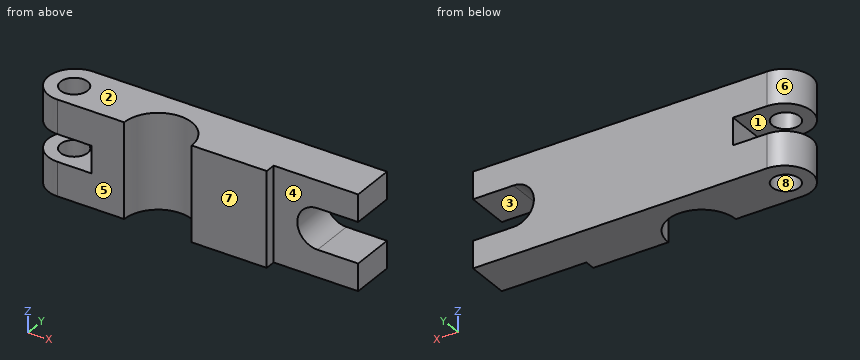
Autodesk Inventor part; units mm, degrees
ref_plane "YZ Plane" through (0, 0, 0) normal (1, 0, 0) x (0, 1, 0)
ref_plane "XZ Plane" through (0, 0, 0) normal (0, 1, 0) x (-1, 0, 0)
ref_plane "XY Plane" through (0, 0, 0) normal (0, 0, 1) x (1, 0, 0)
sketch "Szkic1" plane through (0, 0, 0) normal (0, 0, 1) x (1, 0, 0)
  line L0 (-28.581, 16.053) -> (52, 16.053)
  circle A0 centre (-35, 7.6573) radius 4
  line L1 (52, 16.053) -> (52, 3.053)
  line L2 (52, 3.053) -> (27, 3.053)
  line L3 (27, 3.053) -> (27, -0.0459)
  line L4 (27, -0.0459) -> (4.7982, -0.0459)
  arc A1 (4.7982, -0.0459) -> (-15.2013, 0.053) centre (-5.2013, 0.053) ccw
  line L5 (-28.581, 0.053) -> (-15.2013, 0.053)
  line L6 (-28.581, 0.053) -> (-34.9011, 0.053)
  line L7 (-28.581, 16.053) -> (-34.9011, 16.053)
  arc A2 (-34.9011, 16.053) -> (-34.9011, 0.053) centre (-34.9011, 8.053) ccw
  point P0 (0, 0)
  dimension "d1" = 8
  dimension "d2" = 20
  dimension "d3" = 25
  dimension "d4" = 52
  dimension "d6" = 13
  dimension "d7" = 87
  dimension "d8" = 16
extrude "Wyciągnięcie proste1" add sketch "Szkic1" along normal mid plane 28
sketch "Szkic2" plane through (-34.9011, 16.053, 14) normal (0, 1, 0) x (1, 0, 0)
  line L0 (0, 28) -> (86.9011, 28) construction
  line L1 (86.9011, 0) -> (0, 0) construction
  line L2 (86.9011, 28) -> (86.9011, 0) construction
  line L3 (0, 28) -> (-8, 28) construction
  line L4 (-8, 0) -> (0, 0) construction
  line L5 (-8, 28) -> (-8, 0) construction
  line L6 (-8, 28) -> (-8, 0) construction
  line L7 (-8, 28) -> (-8, 0) construction
  line L8 (-8, 28) -> (-8, 0) construction
  line L9 (-8, 28) -> (-8, 0) construction
  line L10 (-8, 28) -> (-8, 0) construction
  line L11 (-8, 28) -> (-8, 0) construction
  line L12 (-8, 28) -> (-8, 0) construction
  line L13 (-8, 28) -> (-8, 0) construction
  line L14 (-8, 28) -> (-8, 0) construction
  line L15 (-8, 28) -> (-8, 0) construction
  line L16 (-8, 28) -> (-8, 0) construction
  line L17 (-8, 28) -> (-8, 0) construction
  line L18 (-8, 28) -> (-8, 0) construction
  line L19 (0, 28) -> (0, 0) construction
  line L20 (86.9011, 20) -> (74.9011, 20)
  line L21 (86.9011, 8) -> (74.9011, 8)
  arc A0 (74.9011, 20) -> (74.9011, 8) centre (74.9011, 14) ccw
  line L22 (10, 10) -> (10, 18)
  line L23 (10, 18) -> (-8, 18)
  line L24 (3.9011, 0) -> (3.9011, 28)
  line L25 (10, 10) -> (-8, 10)
  line L26 (-8, 18) -> (-8, 10)
  line L27 (86.9011, 20) -> (86.9011, 8)
  point P0 (34.9011, 14)
  dimension "d12" = 12
  dimension "d13" = 40
  dimension "d15" = 8
  dimension "d16" = 18
extrude "Wyciągnięcie proste2" cut sketch "Szkic2" against normal through all
properties part number "Plyta dociskowa"
Verification items for the finished model (mm, model axes). Face numbers are marked on the shaded views. A direction names the side the tool comes from. Coordinates: 2 decimals unless noted, no trailing zeros. Loops run counter-clockwise (first coordinate to the right, second up) from the corner with the lowest first, then second, coordinate; pieces in that order, holes last. Notation, with made-up numbers: (28.25, -11) -> (76.25, -11) arc R20 cw to (76.25, -3) -> close; hole circle Ø9 at (63, 23). An arc over 180 degrees is marked (long way). Answer in a Markdown table with one row per item. Add a question column.
1. Depth check by flat-ended pin: P1, Ø6, axis at y = 11, z = 2, coming from the -X side; P2, Ø2, axis at y = 10.5, z = 4, coming from the +X side; P3, Ø6.5, axis at y = 10.5, z = 0.5, coming from the -X side. Enter the tip coordinate at first touch or a pass-through.
2. Material ranges on probe 1 along Z at (x, y) = (-35.5, 12.75); probe 2 along X at (y, z) = (6.5, -12); probe 3 along X at (y, z) = (4.75, -8), recorded low to high. Write a range as [from, to].
3. Section check C-C, the plane z = -11.5. Enter the section's corners in (x, y).
4. Draft check along Y on the marked faces 6, 7 and 8. Enter one of: +Y half, -Y half, draft (parallel to the pull), parting line (faces both ways), or undercut.
5. Section check A-A, the plane x = 45.5. Enter the section's corners in (y, z).
6. Access from +Z, -Z, +X, -X, +Y, -Y to the whole of each face (thin tool, end or side, straight path). Record for the marked faces 1, 2, 3, 4 and 5.
7. Section check D-D, the plane x = 30. Enter the section's corners in (y, z), then the cut area to 3 significant figures.
8. Section check B-B, the plane z = 0. Enter the section's corners in (x, y), then the cut area to 3 significant figures.
Derived:
| question | item | result |
|---|---|---|
| 1 | P1 | stops at x = -42.87 |
| 1 | P2 | stops at x = 36.68 |
| 1 | P3 | stops at x = -24.9 |
| 2 | probe 1 | z = [-14, -4], [4, 14] |
| 2 | probe 2 | x = [-42.75, -38.83], [-31.17, -12.85], [2.44, 52] |
| 2 | probe 3 | x = [-42.19, -37.75], [-32.25, -14.03], [3.63, 52] |
| 3 | outline | (-34.9, 0.05) -> (-15.2, 0.05) arc R10 cw (long way) to (4.8, -0.05) -> (27, -0.05) -> (27, 3.05) -> (52, 3.05) -> (52, 16.05) -> (-34.9, 16.05) arc R8 ccw to start; hole circle Ø8 at (-35, 7.66) |
| 4 | face 6 | parting line |
| 4 | face 7 | -Y half |
| 4 | face 8 | undercut |
| 5 | outline | (3.05, -14) -> (16.05, -14) -> (16.05, -6) -> (3.05, -6) -> close; (3.05, 6) -> (16.05, 6) -> (16.05, 14) -> (3.05, 14) -> close |
| 6 | face 1 | -X, +Y, -Y |
| 6 | face 2 | +Z, +X, -X, +Y, -Y |
| 6 | face 3 | +X, +Y, -Y |
| 6 | face 4 | +Z, -Z, +X, -Y |
| 6 | face 5 | +Z, -Z, -X, -Y |
| 7 | outline | (3.05, -14) -> (16.05, -14) -> (16.05, 14) -> (3.05, 14) -> close |
| 7 | area | 364 mm² |
| 8 | outline | (-24.9, 0.05) -> (-15.2, 0.05) arc R10 cw (long way) to (4.8, -0.05) -> (27, -0.05) -> (27, 3.05) -> (34, 3.05) -> (34, 16.05) -> (-24.9, 16.05) -> close |
| 8 | area | 767 mm² |
